```python
from build123d import *

# Parameters (mm, degrees)
CROQUIS2_W                   = 120
CROQUIS2_H                   = 45
SALIENTE_EXTRUIR1_DEPTH      = 5
SALIENTE_EXTRUIR1_DEPTH_BACK = 45
VACIADO1_T                   = -3
CORTAR_EXTRUIR2_START        = -10.5
CORTAR_EXTRUIR2_DEPTH        = 10.5
CORTAR_EXTRUIR3_REACH        = 122
CROQUIS4_R                   = 1.55
CROQUIS4_W                   = 8
CROQUIS4_H                   = 10.5
CORTAR_EXTRUIR4_REACH        = 52
CROQUIS5_R                   = 1.55


with BuildPart() as part:
    # Croquis2 → Saliente-Extruir1 (new body, two sides)
    with BuildSketch(Plane.XY.offset(-12)) as saliente_extruir1_sk:
        with Locations((0, -53.288987008)):
            Rectangle(CROQUIS2_W, CROQUIS2_H)
    extrude(amount=SALIENTE_EXTRUIR1_DEPTH)
    extrude(saliente_extruir1_sk.sketch, amount=-SALIENTE_EXTRUIR1_DEPTH_BACK)

    # Vaciado1
    vaciado1_openings = [part.faces().sort_by_distance(p)[0] for p in [
        (0, -75.788987008, -32),
    ]]
    offset(amount=VACIADO1_T, openings=vaciado1_openings, kind=Kind.INTERSECTION)

    # Croquis3 → Cortar-Extruir2 (cut)
    with BuildSketch(Plane.XY.offset(-7).offset(CORTAR_EXTRUIR2_START)):
        Polygon((0, 88.470820393), (-19.862936734, 27.338987008), (-84.140750237, 27.338987008), (-32.138906752, -10.442563819), (-52.001843485, -71.574397204), (0, -33.792846378), (52.001843485, -71.574397204), (32.138906752, -10.442563819), (84.140750237, 27.338987008), (19.862936734, 27.338987008), align=None)
    extrude(amount=CORTAR_EXTRUIR2_DEPTH, mode=Mode.SUBTRACT)

    # Croquis4 → Cortar-Extruir3 (cut, up to next)
    with BuildSketch(Plane.ZY.offset(60), mode=Mode.PRIVATE) as cortar_extruir3_sk1:
        with Locations((-43.35, -37.771593165)):
            Circle(CROQUIS4_R)
    cortar_extruir3_tool1 = extrude(cortar_extruir3_sk1.sketch, amount=-CORTAR_EXTRUIR3_REACH, mode=Mode.PRIVATE) & part.part
    add(cortar_extruir3_tool1.solids().sort_by_distance((-60, -37.771593, -43.35))[0], mode=Mode.SUBTRACT)
    # Croquis4 → Cortar-Extruir3 (cut, up to next)
    with BuildSketch(Plane.ZY.offset(60), mode=Mode.PRIVATE) as cortar_extruir3_sk2:
        with Locations((-43.35, -68.73680548)):
            Circle(CROQUIS4_R)
    cortar_extruir3_tool2 = extrude(cortar_extruir3_sk2.sketch, amount=-CORTAR_EXTRUIR3_REACH, mode=Mode.PRIVATE) & part.part
    add(cortar_extruir3_tool2.solids().sort_by_distance((-60, -68.736805, -43.35))[0], mode=Mode.SUBTRACT)
    # Croquis4 → Cortar-Extruir3 (cut, up to next)
    with BuildSketch(Plane.ZY.offset(60), mode=Mode.PRIVATE) as cortar_extruir3_sk3:
        with Locations((-48.5, -53.254199323)):
            Rectangle(CROQUIS4_W, CROQUIS4_H)
    cortar_extruir3_tool3 = extrude(cortar_extruir3_sk3.sketch, amount=-CORTAR_EXTRUIR3_REACH, mode=Mode.PRIVATE) & part.part
    add(cortar_extruir3_tool3.solids().sort_by_distance((-60, -53.254199, -48.5))[0], mode=Mode.SUBTRACT)

    # Croquis5 → Cortar-Extruir4 (cut, up to next)
    with BuildSketch(Plane(origin=(0, 0, -57), x_dir=(-1, 0, 0), z_dir=(0, 0, -1)), mode=Mode.PRIVATE) as cortar_extruir4_sk1:
        with Locations((7.617393842, -53.254199323)):
            Circle(CROQUIS5_R)
    cortar_extruir4_tool1 = extrude(cortar_extruir4_sk1.sketch, amount=-CORTAR_EXTRUIR4_REACH, mode=Mode.PRIVATE) & part.part
    add(cortar_extruir4_tool1.solids().sort_by_distance((-7.617394, -53.254199, -57))[0], mode=Mode.SUBTRACT)


solid = part.part
```
Source: CAD feature listing. Evaluate the final solid. Frame: model axes, mm. A direction names the side the tool comes from. Give positions to 0.01 mm unless a question says otherwise; leave off trailing zeros. Order: outer loops, then holes, each group sorted by start corner. A loop starts at its lowest first (then second) coordinate and runs counter-clockwise, first axis right, second up.
(1) Contact query for flat-ended pins moving along their axis: P1, Ø22, axis at x = 9, z = -28, coming from the -Y side; P2, Ø3, axis at y = -37.77, z = -43.35, coming from the -X side; P3, Ø1.5, axis at x = 15.5, z = -12, coming from the +Y side; P4, Ø1.5, axis at x = -16.5, y = -32.5, coming from the +Z side. Output: stop coordinate, or through.
(2) Material intervals for line 1 along X through (y, z) = (-62, -46); line 2 along Z through (x, y) = (-49, -71.5); line 3 along Y through (x, z) = (-59, -43), sorted ascending.
(3) Section query D-D (z = -13). Return the cut outline in (x, y).
(4) Pull-direction query (Y, two-part tool) for faces 4 (the face through (-1, -59, -10)), 5 (the face through (0, -75.789, -56)), 6 (the face through (-26.365, -52.948, -8.521)); classes: +Y half, -Y half, draft (parallel to the pull), parting line (faces both ways), or undercut.
(5) Section query C-C (z = -38). Return the cut outline in (x, y).
(6) Section query B-B (x = 4). Return the cut outline in (y, z).
(7) Access query for faces 1 (the face through (-59, -58.504, -49)), 2 (the face through (-1, -33.789, -37)), 3 (the face through (43.996, -46.935, -8.824)). Directions: +Z, -Z, +X, -X, +Y, -Y. A direction counts if a zero-diameter tool reaches every point of the face in a straight line with its end or side. Return the directions, or none.
(8) Section query A-A (z = -48). Return the cut outline in (x, y), plus the area to 4 significant figures.
Outcome:
1. P1: stops at y = -33.79
1. P2: stops at x = 57
1. P3: passes through
1. P4: stops at z = -17.5
2. line 1: x = -60 to -57, 57 to 60
2. line 2: z = -57 to -54, -10 to -7
2. line 3: y = -75.79 to -70.25, -67.23 to -39.28, -36.26 to -30.79
3. outline: (-60, -75.79) - (-57, -75.79) - (-57, -33.79) - (-39.72, -33.79) - (-38.75, -30.79) - (-60, -30.79) - close; (38.75, -30.79) - (39.72, -33.79) - (57, -33.79) - (57, -75.79) - (60, -75.79) - (60, -30.79) - close
4. face 4: draft
4. face 5: -Y half
4. face 6: undercut
5. outline: (-60, -75.79) - (-57, -75.79) - (-57, -33.79) - (57, -33.79) - (57, -75.79) - (60, -75.79) - (60, -30.79) - (-60, -30.79) - close
6. outline: (-75.79, -57) - (-30.79, -57) - (-30.79, -17.5) - (-33.79, -17.5) - (-33.79, -54) - (-75.79, -54) - close; (-75.79, -10) - (-36.7, -10) - (-36.7, -7) - (-75.79, -7) - close
7. face 1: -X
7. face 2: -Y
7. face 3: +Z
8. outline: (-60, -75.79) - (-57, -75.79) - (-57, -58.5) - (-60, -58.5) - close; (-60, -48) - (-57, -48) - (-57, -33.79) - (57, -33.79) - (57, -75.79) - (60, -75.79) - (60, -30.79) - (-60, -30.79) - close
8. area: 580.5 mm2
